Check sheet for the modelled part. Datum: model origin and axes. Units: mm. Face numbers are marked on the shaded views. A direction names the side the tool comes from. Round coordinates to 2 decimals unless told otherwise and drop trailing zeros. Loops run counter-clockwise (first coordinate to the right, second up) from the corner with the lowest first, then second, coordinate; pieces in that order, holes last. Notation, with made-up numbers: (74, 64) - (115, 64) arc R17 cw to (115, 79) - close; hole circle Ø1 at (87, 89). An arc over 180 degrees is marked (long way). Put each result on its own line as item: value.
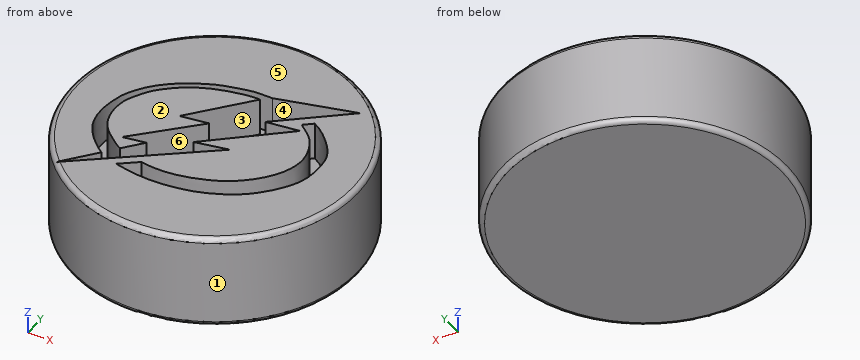
```python
from build123d import *

# Parameters (mm, degrees)
F0_R     = 38.1
F1_DEPTH = 25.4
F2_R     = 1.27
F4_DEPTH = 10.16


with BuildPart() as f1:
    # F0 (on Top) → F1 (new body)
    with BuildSketch(Plane.XY):
        Circle(F0_R)
    extrude(amount=F1_DEPTH)

    # F2
    f2_edges = [f1.edges().sort_by_distance(p)[0] for p in [
        (-38.1, 0, 25.4),
        (-38.1, 0, 0),
    ]]
    fillet(f2_edges, radius=F2_R)

    # F3 (on face) → F4 (cut)
    with BuildSketch(Plane.XY.offset(25.4)):
        with BuildLine():
            Line((-19.5661182899, -18.1706012091), (-26.7553265637, -26.4851974048))
            Line((-26.7553265637, -26.4851974048), (5.4061874503, -2.5106431912))
            Line((5.4061874503, -2.5106431912), (-3.200049929, -4.2408025526))
            Line((-3.200049929, -4.2408025526), (15.8394873054, 11.5967263231))
            Line((15.8394873054, 11.5967263231), (7.2614595686, 10.4792513123))
            Line((7.2614595686, 10.4792513123), (24.433595378, 24.2147761598))
            Line((24.433595378, 24.2147761598), (4.2949300972, 18.9045294))
            add(Edge.make_bspline(
                [(4.2949300972, 18.9045294), (3.8578868072, 18.9001902263), (2.8255551255, 18.8899407461), (0.0728269951, 18.9879537596), (-2.416985134, 18.5661852441), (-6.4107369283, 17.6468576464), (-9.7123233005, 16.7021829393), (-12.5398092723, 15.3440163882), (-16.8721606771, 13.1040275758), (-19.9007344343, 10.7357054975), (-22.8894463137, 8.0049544035), (-25.8325272327, 3.571514678), (-26.5942743919, 1.0228501359), (-27.8243775869, -3.8193612894), (-27.1445214519, -10.193277819), (-23.7350134876, -14.6357550528), (-21.4008680736, -16.806202139), (-20.1406895566, -17.7433252345), (-19.5661182899, -18.1706012091)],
                knots=[0, 0, 0, 0, 0.0393230905, 0.0928843277, 0.1459402353, 0.2120782925, 0.2727584507, 0.3308515796, 0.40286638, 0.4671851532, 0.533772906, 0.608108541, 0.6617575665, 0.7335395787, 0.8165602186, 0.8932761667, 0.9513398719, 1, 1, 1, 1], degree=3))
        make_face()
        with BuildLine():
            add(Edge.make_bspline(
                [(2.0359272731, 17.0305203597), (1.3954106628, 17.0546042076), (-0.0892415224, 17.1104281111), (-3.5731065553, 16.5502831509), (-8.5082169393, 15.40758038), (-12.1799994257, 13.8781536445), (-15.6913864649, 12.0326267348), (-18.7093375005, 9.6369774455), (-21.4249459198, 7.0615317926), (-23.465217898, 3.5036235622), (-24.8205084542, 1.0789665507), (-25.414591442, -3.8024334011), (-23.9169773543, -8.8156140602), (-20.9006750006, -11.7286450069), (-17.920148096, -14.0343436431), (-17.0053674551, -14.5514987399), (-16.6593735189, -14.7471003077)],
                knots=[0, 0, 0, 0, 0.0533585134, 0.1236795927, 0.2084451349, 0.2836295249, 0.3576121735, 0.4308488556, 0.5037700814, 0.5784669466, 0.6408484233, 0.7223586051, 0.8071746244, 0.8844167139, 0.9562833817, 1, 1, 1, 1], degree=3))
            Line((2.0359272731, 17.0305203597), (-10.8908848154, 2.4554725062))
            Line((-10.8908848154, 2.4554725062), (-3.5924285351, 3.5412959569))
            Line((-3.5924285351, 3.5412959569), (-18.3622744366, -10.8986072092))
            Line((-18.3622744366, -10.8986072092), (-12.4181416451, -9.8916973697))
            Line((-12.4181416451, -9.8916973697), (-16.6593735189, -14.7471003077))
        make_face(mode=Mode.SUBTRACT)
        with BuildLine():
            add(Edge.make_bspline(
                [(17.3873861626, 15.6334186555), (18.0370958634, 15.2589721072), (19.3749563206, 14.4879243151), (21.3265644237, 12.8038361847), (23.0478327612, 10.9995316669), (24.778719369, 8.9559550933), (26.2146688484, 6.1020958965), (26.3979131008, 3.9139763932), (26.5491055591, 2.71825424), (26.4625942606, -0.8082938445), (25.5136962919, -4.8925023756), (22.5000147718, -9.5825463131), (17.5963832254, -14.740520896), (12.3872032479, -17.7055628688), (7.5630660017, -19.7133836725), (3.1258890287, -20.746211478), (-2.1365566408, -21.5172519141), (-8.365474944, -21.4265742118), (-12.4795067403, -20.5878213551), (-14.5448679776, -20.1667435114)],
                knots=[0, 0, 0, 0, 0.0448250287, 0.092302198, 0.1390260415, 0.1877941832, 0.2409788153, 0.2837285607, 0.3160106559, 0.3702840764, 0.4314149985, 0.501108459, 0.5803195518, 0.6531562215, 0.7203239803, 0.783247441, 0.851372124, 0.9253845694, 1, 1, 1, 1], degree=3))
            Line((17.3873861626, 15.6334186555), (15.0031798623, 13.7454713383))
            add(Edge.make_bspline(
                [(-9.8547809612, -16.6705540785), (-8.8513922673, -16.8368529644), (-6.6835445534, -17.1961460894), (-2.2683618168, -17.0786395481), (1.9592718785, -16.373668921), (8.3191866593, -14.3188597994), (12.4218579634, -12.0285396002), (16.7822239361, -8.3732731196), (20.3852473964, -3.7979371357), (22.5516095847, 2.5973484144), (20.2177525614, 9.1228571556), (17.816185371, 11.551632666), (15.9466715379, 13.0096503389), (15.0031798623, 13.7454713383)],
                knots=[0, 0, 0, 0, 0.0734379394, 0.1586646033, 0.2453518248, 0.3507074217, 0.4408496419, 0.5375155853, 0.636853644, 0.7423131031, 0.8474861883, 0.9230305178, 1, 1, 1, 1], degree=3))
            Line((-9.8547809612, -16.6705540785), (-14.5448679776, -20.1667435114))
        make_face()
    extrude(amount=-F4_DEPTH, mode=Mode.SUBTRACT)


solid = f1.part
```
Item 1: Section check A-A on z = 21.25. Count the separate pieces of the cut face and the enclosed holes in it, then the cut area to 3 significant figures.
Filled sheet:
separate pieces: 2
enclosed holes: 2
area: 3,660 mm²
Item 2: Section check B-B on z = 12.25. Enter the section's corners in (x, y), then the cut area to 3 significant figures.
Filled sheet:
outline: circle Ø76.2 at (0, 0)
area: 4,560 mm²
Item 3: Tool access check on the marked faces 5 and 6. Record the directions out of +Z, -Z, +X, -X, +Y, -Y that give a thin tool (end or side, any length) a straight path to the whole face; none if there is none.
Filled sheet:
face 5: +Z, +X, -X, +Y, -Y
face 6: +Z
Item 4: Go/stop test with flat-tipped pins: pin 1 (3 mm diameter, centred on y = 10.5, z = 4, fed in from -X); pin 2 (1.5 mm diameter, centred on y = 8.5, z = 7.5, fed in from -X); pin 3 (1 mm diameter, centred on x = -8.5, z = 22, fed in from -Y). Record where each tip stops, or that it passes through.
Filled sheet:
pin 1: x = -37.02
pin 2: x = -37.3
pin 3: y = -37.25
Item 5: Thickness scan on line 1 (X direction, y = 4, z = 21.5); line 2 (Y direction, x = 23.5, z = 16); line 3 (Y direction, x = 22, z = 17.25). Record the ranges inside material, lowest first. Write a range as from..to.
Filled sheet:
line 1: -37.89..-25.41, -23.18..-9.52, 6.71..21.64, 26.4..37.89
line 2: -29.99..-7.89, 10.45..23.47, 23.97..29.99
line 3: -31.11..-9.88, 12.08..22.27, 23.57..31.11
Item 6: Release check for a two-part mould opening along Y. For the marked faces 1, 2, 3 and 4 record: +Y half, -Y half, draft (parallel to the pull), parting line (faces both ways), or undercut.
Filled sheet:
face 1: parting line
face 2: draft
face 3: undercut
face 4: undercut
